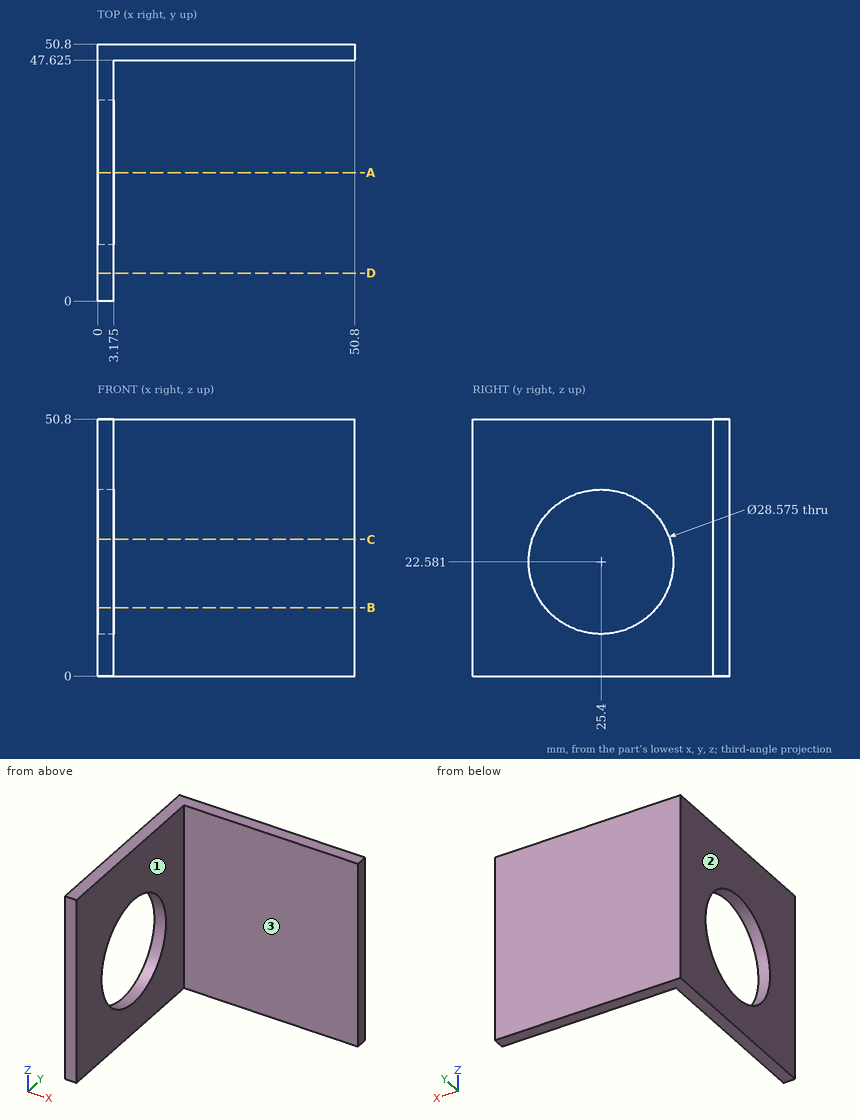
Source: three-view drawing plus pictorial views. Frame: mm from the lowest corner of the part. Coordinates: 2 decimals unless noted, no trailing zeros. Loops run counter-clockwise (first coordinate to the right, second up) from the corner with the lowest first, then second, coordinate; pieces in that order, holes last. Notation, with made-up numbers: (42, 51.5) - (99, 51.5) arc R29 ccw to (99, 76.5) - close; hole circle Ø11 at (12.5, 52). An arc over 180 degrees is marked (long way). One line per question, with ' | ' between items.
1) Section D-D, the plane y = 5.5. Return loops of the section in (x, z) (1 decimal), then the cut area to 3 significant figures.
Report:
outline: (0, 0) - (3.2, 0) - (3.2, 50.8) - (0, 50.8) - close | area: 161 mm²
2) Pull-direction query (X, two-part tool) for the marked faces 1, 2 and 3; classes: released by +X, released by -X, zero draft, split by the parting line, or undercut.
Report:
face 1: released by +X | face 2: released by -X | face 3: zero draft
3) Line query: line 1 along Y through (x, z) = (8, 30) (1 decimal); line 2 along X through (y, z) = (46.5, 19.5) (1 decimal). Output: solid intervals per line, ascending.
Report:
line 1: y = 47.6 to 50.8 | line 2: x = 0 to 3.2
4) First-contact query: P1, Ø4, axis at x = 14.5, z = 25, coming from the -Y side (3 decimals); P2, Ø5, axis at y = 9.5, z = 25, coming from the +X side (3 decimals). Flat tips, straight axial feed; report the tip coordinate or a pass-through.
Report:
P1: stops at y = 47.625 | P2: stops at x = 3.175
5) Section C-C, the plane z = 27. Return loops of the section in (x, y) (1 decimal), then the cut area to 3 significant figures.
Report:
outline: (0, 0) - (3.2, 0) - (3.2, 11.8) - (0, 11.8) - close; (0, 39) - (3.2, 39) - (3.2, 47.6) - (50.8, 47.6) - (50.8, 50.8) - (0, 50.8) - close | area: 226 mm²
6) Section B-B, the plane z = 13.5. Return loops of the section in (x, y) (1 decimal).
Report:
outline: (0, 0) - (3.2, 0) - (3.2, 14.4) - (0, 14.4) - close; (0, 36.4) - (3.2, 36.4) - (3.2, 47.6) - (50.8, 47.6) - (50.8, 50.8) - (0, 50.8) - close
7) Section A-A, the plane y = 25.4. Return loops of the section in (x, z) (1 decimal).
Report:
outline: (0, 0) - (3.2, 0) - (3.2, 8.3) - (0, 8.3) - close; (0, 36.9) - (3.2, 36.9) - (3.2, 50.8) - (0, 50.8) - close
